Autodesk Fusion 360 part; units mm, degrees
sketch "Skizze1" plane through (0, 0, 0) normal (1, 0, 0) x (0, 0, -1)
  line L0 (-13, 0) -> (-13, 19)
  line L1 (-11.18, 17.291) -> (-11.18, 0)
  line L2 (-11.18, 0) -> (-13, 0)
  line L3 (0, 0) -> (-7.615, 0)
  line L4 (-7.615, 0) -> (-6.5, 0)
  line L5 (-7.615, 0) -> (-7.615, 17)
  line L6 (-7.615, 17) -> (-11.18, 17)
  line L7 (-6.5, 0) -> (-6.5, 20)
  line L8 (0, 0) -> (0, 53.458)
  line L9 (-6.5, 20) -> (-5, 35)
  line L10 (-11, 60) -> (-11, 43)
  line L11 (-13, 19) -> (-13, 19.5458)
  line L12 (-11, 60) -> (-9, 60)
  line L13 (-9, 60) -> (-9, 42)
  arc A0 (-5, 39) -> (-8, 42) centre (-8.5, 38.5) ccw
  line L14 (-9, 42) -> (-8, 42)
  line L15 (-5, 39) -> (-5, 35)
  line L16 (-12.7481, 20.3779) -> (-11, 23)
  line L17 (-11, 23) -> (-9.2519, 25.6221)
  line L18 (-9, 26.4542) -> (-9, 37)
  line L19 (-11, 43) -> (-11, 41.6213)
  line L20 (-10.5607, 40.5607) -> (-9.4393, 39.4393)
  line L21 (-9, 38.3787) -> (-9, 37)
  arc A1 (-11, 41.6213) -> (-10.5607, 40.5607) centre (-9.5, 41.6213) ccw
  arc A2 (-9, 38.3787) -> (-9.4393, 39.4393) centre (-10.5, 38.3787) ccw
  arc A3 (-9.2519, 25.6221) -> (-9, 26.4542) centre (-10.5, 26.4542) ccw
  arc A4 (-12.7481, 20.3779) -> (-13, 19.5458) centre (-11.5, 19.5458) ccw
  dimension "d3" = 7.615
  dimension "d4" = 1.115
  dimension "d7" = 1.5
revolve "Drehen1" add sketch "Skizze1" angle 360 about axis through (0, 0, 0) along (0, 1, 0)
hole "Bohrung1" at (0, 36.7372, 9) direction (0, 0, -1) diameter 2 depth 9 tip angle 118
hole "Bohrung2" at (0, 43.5811, 11) direction (0, 0, -1) diameter 2 depth 9 tip angle 118
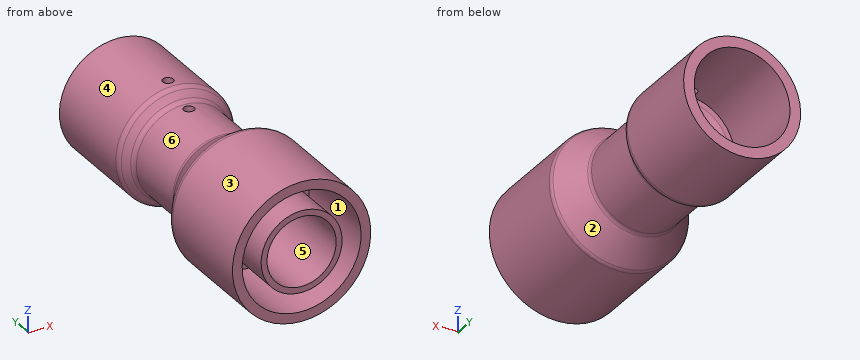
Geometry check sheet. Reference: the model listing, model coordinates, mm. Face numbers are marked on the shaded views. A direction names the side the tool comes from. Round coordinates to 2 decimals unless told otherwise and drop trailing zeros. Loops run counter-clockwise (first coordinate to the right, second up) from the corner with the lowest first, then second, coordinate; pieces in that order, holes last. Notation, with made-up numbers: (69.5, 69) - (79.5, 69) arc R19 cw to (79.5, 91) - close; hole circle Ø4 at (2, 80.25). An arc over 180 degrees is marked (long way). Write each question's results on one line, items separated by ' | '. Start each with the question number.
Q1. Gauge pin test, flat ends, axial feed: P1, Ø12, axis at x = -8, y = 33.5, coming from the +Z side; P2, Ø12, axis at x = 2.5, z = -1.5, coming from the +Y side; P3, Ø1, axis at x = -7.5, y = 47, coming from the -Z side. Record the tip position at first contact, or that the pin passes through.
Q2. Cross-section at A-A on y = 54. Enter the section's corners in (x, z).
Q3. Release check for a two-part mould opening along X. For the marked faces 1 and 2 record: +X half, -X half, draft (parallel to the pull), parting line (faces both ways), or undercut.
Q4. Cross-section at C-C on y = 28. Enter the section's corners in (x, z).
Q5. Access from +Z, -Z, +X, -X, +Y, -Y to the whole of each face (thin tool, end or side, straight path). Record for the marked faces 3, 4, 5 and 6.
Q6. Thickness scan on line 1 (X direction, y = 7.5, z = 0) (3 decimals); line 2 (Z direction, x = -0.25, y = 52.5); line 3 (Y direction, x = 0, z = 6.85). Record the ranges inside material, lowest first. Write a range as [from, to].
Q7. Cross-section at B-B on x = 0. State how many separate pieces and enclosed holes the cut face has, and give its area (3 significant figures).
Answers below:
1) P1: stops at z = 8.77 | P2: stops at y = 42 | P3: stops at z = -8.49
2) outline: circle Ø22 at (0, 0); hole circle Ø18 at (0, 0)
3) face 1: undercut | face 2: parting line
4) outline: circle Ø18 at (0, 0); hole circle Ø11.4 at (0, 0)
5) face 3: +Y, -Y | face 4: +Y | face 5: -Y | face 6: none
6) line 1: x = [-13, -11.18], [-7.615, -6.5], [6.5, 7.615], [11.18, 13] | line 2: z = [-11, -9], [9, 11] | line 3: y = [0, 35.74], [37.74, 41.63]
7) separate pieces: 4 | enclosed holes: 0 | area: 379 mm²
